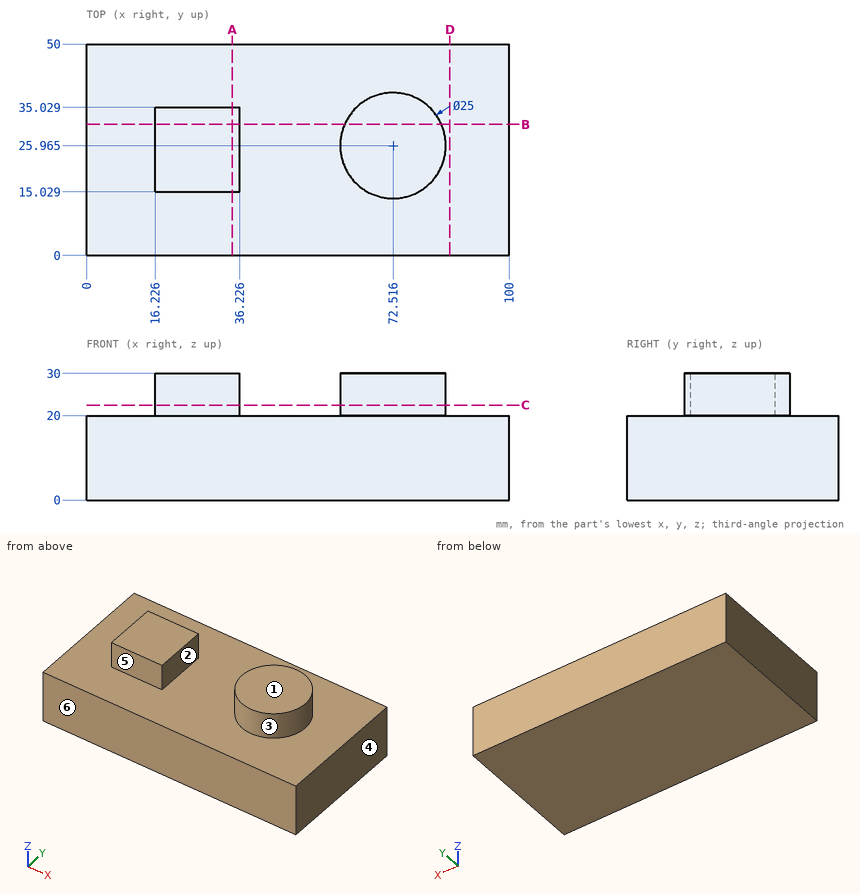
Answer from the drawing. Dimensions are ordinates in mm from the lowest x, y and z of the part. A direction names the side the tool comes from. Give positions to 0.01 mm unless a question says otherwise; leave off trailing zeros. Order: outer loops, then holes, each group sorted by start corner. A loop starts at its lowest first (then second) coordinate and runs counter-clockwise, first axis right, second up. Notation, with made-up numbers: (-4, 35) - (6, 35) arc R27 cw to (6, 73) - close; hole circle Ø6 at (-24.5, 52.25). An arc over 180 degrees is marked (long way). Use one line per item in the form item = value.
1) Find section B-B on y = 31. Determine the outline of the cut face in (x, z) (1 decimal).
Verdict:
outline = (0, 0) - (100, 0) - (100, 20) - (84, 20) - (84, 30) - (61.1, 30) - (61.1, 20) - (36.2, 20) - (36.2, 30) - (16.2, 30) - (16.2, 20) - (0, 20) - close
2) The mould has two halves that part along X. Classify the marked faces 1, 2, 3 and 4: released by +X, released by -X, zero draft, split by the parting line, or undercut.
Verdict:
face_1 = zero draft
face_2 = undercut
face_3 = undercut
face_4 = released by +X
3) Consider probe 1 along Z at (x, y) = (7, 41); probe 2 along X at (y, z) = (22.5, 22) (1 decimal); probe 3 along Y at (x, z) = (21.5, 27.25). Determine where each line is inside the solid, lowest interval first. Write a range as [from, to].
Verdict:
probe_1 = [0, 20]
probe_2 = [16.2, 36.2], [60.5, 84.5]
probe_3 = [15.03, 35.03]
4) Find section A-A on x = 34.5. Determine the outline of the cut face in (y, z), and give its area (3 significant figures).
Verdict:
outline = (0, 0) - (50, 0) - (50, 20) - (35.03, 20) - (35.03, 30) - (15.03, 30) - (15.03, 20) - (0, 20) - close
area = 1,200 mm^2
5) Find section C-C on z = 22.5. Determine the outline of the cut face in (x, y) (1 decimal), and give its area (3 significant figures).
Verdict:
outline = (16.2, 15) - (36.2, 15) - (36.2, 35) - (16.2, 35) - close; circle Ø25 at (72.5, 26)
area = 891 mm^2
6) Find section D-D on x = 86. Determine the outline of the cut face in (y, z), and give its area (3 significant figures).
Verdict:
outline = (0, 0) - (50, 0) - (50, 20) - (0, 20) - close
area = 1,000 mm^2
7) Each of these flat-tipped pins is pushed along its axis until it touches: pin 1 (3 mm diameter, centred on x = 30, z = 27.5, fed in from -Y); pin 2 (5 mm diameter, centred on y = 24, z = 24, fed in from +X); pin 3 (5 mm diameter, centred on y = 23, z = 25, fed in from -X). Where does it stop, or does it pass through?
Verdict:
pin_1 = 15.03
pin_2 = 85.02
pin_3 = 16.23
8) For the marked faces 5 and 6, determine the directions among +Z, -Z, +X, -X, +Y, -Y from which every point of the face is accessible in a straight line to the end or side of a thin tool.
Verdict:
face_5 = +Z, -X, -Y
face_6 = +Z, -Z, +X, -X, -Y
